```python
from build123d import *

# Parameters (mm, degrees)
CROQUIS1_W               = 180
CROQUIS1_H               = 140
SALIENTE_EXTRUIR1_DEPTH  = 80
CROQUIS2_W               = 12
CROQUIS2_H               = 140
SALIENTE_EXTRUIR2_DEPTH  = 3
REDONDEO1_R              = 5
CROQUIS3_R               = 2.5
CORTAR_EXTRUIR1_DEPTH    = 4
REDONDEO1_OF_SIMETR_A1_R = 5
REDONDEO2_R              = 10


with BuildPart() as part:
    # Croquis1 → Saliente-Extruir1 (new body)
    with BuildSketch(Plane(origin=(0, 0, 0), x_dir=(1, 0, 0), z_dir=(0, 1, 0))):
        Rectangle(CROQUIS1_W, CROQUIS1_H)
    extrude(amount=SALIENTE_EXTRUIR1_DEPTH)

    # Croquis2 → Saliente-Extruir2 (add)
    with BuildSketch(Plane.XZ):
        with Locations((96, 0)):
            Rectangle(CROQUIS2_W, CROQUIS2_H)
    saliente_extruir2 = extrude(amount=-SALIENTE_EXTRUIR2_DEPTH)

    # Redondeo1
    redondeo1_edges = [part.edges().sort_by_distance(p)[0] for p in [
        (102, 1.5, 70),
        (102, 1.5, -70),
    ]]
    fillet(redondeo1_edges, radius=REDONDEO1_R)

    # Croquis3 → Cortar-Extruir1 (cut, through all)
    with BuildSketch(Plane(origin=(0, 3, 0), x_dir=(1, 0, 0), z_dir=(0, 1, 0))):
        with Locations((97, 50)):
            Circle(CROQUIS3_R)
        with Locations((97, -50)):
            Circle(CROQUIS3_R)
    cortar_extruir1 = extrude(amount=-CORTAR_EXTRUIR1_DEPTH, mode=Mode.SUBTRACT)

    # Simetría1: Saliente-Extruir2, Cortar-Extruir1 across plane
    add(saliente_extruir2.mirror(Plane(origin=(0, 0, 0), x_dir=(0, 0, 1), z_dir=(1, 0, 0))))
    add(cortar_extruir1.mirror(Plane(origin=(0, 0, 0), x_dir=(0, 0, 1), z_dir=(1, 0, 0))), mode=Mode.SUBTRACT)

    # Redondeo1 of Simetría1
    redondeo1_of_simetr_a1_edges = [part.edges().sort_by_distance(p)[0] for p in [
        (-102, 1.5, 70),
        (-102, 1.5, -70),
    ]]
    fillet(redondeo1_of_simetr_a1_edges, radius=REDONDEO1_OF_SIMETR_A1_R)

    # Redondeo2
    redondeo2_edges = [part.edges().sort_by_distance(p)[0] for p in [
        (0, 80, 70),
        (0, 80, -70),
    ]]
    fillet(redondeo2_edges, radius=REDONDEO2_R)


solid = part.part
```
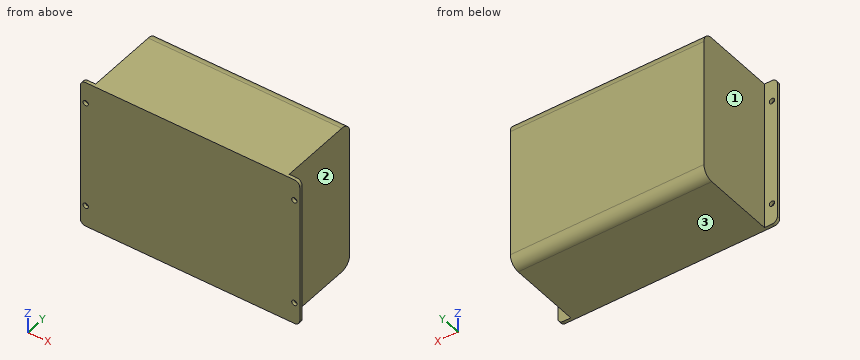
The listing builds one solid part. Answer for the finished solid, in the listing's coordinates (mm). Face numbers are marked on the shaded views. A direction names the side the tool comes from. Give positions to 0.01 mm unless a question says otherwise; leave off trailing zeros. Loops run counter-clockwise (first coordinate to the right, second up) from the corner with the lowest first, then second, coordinate; pieces in that order, holes last. Notation, with made-up numbers: (-25, -13) - (8, -13) arc R20 ccw to (8, 10) - close; hole circle Ø11 at (78, 88.5). An arc over 180 degrees is marked (long way). Return JSON: item names as keys, results as strings. Group by question number.
1. Find section C-C (y = 29). Write down the section's boundary in (x, z).
2. Find section A-A (z = -50). Write down the section's boundary in (x, y), then the cut area to 3 significant figures.
3. Which of the six approach directions +Z, -Z, +X, -X, +Y, -Y give full straight-line access (tool end or side, diameter ignored) to the marked faces 1, 2 and 3?
4. Find section B-B (z = 41). Write down the section's boundary in (x, y).
5. Given pin 1 Ø4 at (y, z) = (34, -42) entering from -X; pin 2 Ø6.5 at (x, z) = (97, 50) entering from +Y; pin 3 Ø10 at (y, z) = (44, -53) entering from +X, each flat-ended and moving along its own axis, determine where each tip first touches the part or whether it passes through.
6. Straight lines are drawn through the part: line 1 (Z direction, x = 97, y = 1.95); line 2 (X direction, y = 1.5, z = 50); line 3 (X direction, y = 60.5, z = -55.5). For each, find the intervals that lie inside material, in ascending order. Write a range as [from, to].
7. Find section D-D (y = 72.5). Write down the section's boundary in (x, z), then the cut area to 3 significant figures.
Verdict:
{
 "1": {"outline": "(-90, -70) - (90, -70) - (90, 70) - (-90, 70) - close"},
 "2": {"outline": "(-102, 0) - (-99.5, 0) - (-99.5, 3) - (-102, 3) - close; (-94.5, 0) - (94.5, 0) - (94.5, 3) - (90, 3) - (90, 80) - (-90, 80) - (-90, 3) - (-94.5, 3) - close; (99.5, 0) - (102, 0) - (102, 3) - (99.5, 3) - close", "area": "14,400 mm^2"},
 "3": {"face 1": "+Z, -Z, -X, +Y", "face 2": "+Z, -Z, +X, +Y", "face 3": "-Z, +X, -X, +Y, -Y"},
 "4": {"outline": "(-102, 0) - (102, 0) - (102, 3) - (90, 3) - (90, 80) - (-90, 80) - (-90, 3) - (-102, 3) - close"},
 "5": {"pin 1": "stops at x = -90", "pin 2": "stops at y = 3", "pin 3": "stops at x = 90"},
 "6": {"line 1": "z = [-70, -52.5], [-47.5, 47.5], [52.5, 70]", "line 2": "x = [-102, -99.5], [-94.5, 94.5], [99.5, 102]", "line 3": "x = [-90, 90]"},
 "7": {"outline": "(-90, -69.68) - (90, -69.68) - (90, 69.68) - (-90, 69.68) - close", "area": "25,100 mm^2"}
}
